For this review, take the finished solid that the model builds, in its own axes (mm). A direction names the side the tool comes from. Coordinates: 2 decimals unless noted, no trailing zeros. Write each loop counter-clockwise with the first axis right and the second up, starting at its lowest first coordinate (ties: lowest second). Pieces come first, ordered by that corner, then holes.
```python
from build123d import *

# Parameters (mm, degrees)
F1_DEPTH = 25.4


with BuildPart() as f1:
    # F0 (on Top) → F1 (new body)
    with BuildSketch(Plane.XY):
        Polygon((-8.610348, -27.288182), (-4.851862, -27.620565), (-4.851862, -13.374916), (-24.708377, -13.374916), (-26.625844, -15.89603), align=None)
        Polygon((-4.851862, -13.374916), (-4.851862, -27.620565), (10.862285, -29.010251), (23.049237, -11.922023), (15.101224, 10.597347), (-5.166208, 12.319417), (-24.708377, -13.374916), align=None)
        Polygon((-30.251862, -13.374916), (-30.251862, -38.774916), (-4.851862, -38.774916), (-4.851862, -27.620565), (-8.610348, -27.288182), (-26.625844, -15.89603), (-24.708377, -13.374916), align=None)
    extrude(amount=F1_DEPTH)


solid = f1.part
```
Q1. For probe 1 along Y at (x, z) = (-26.5, 15.25); probe 2 along X at (y, z) = (-35, 19.5); probe 3 along X at (y, z) = (10, 2.75), list the stretches that pass through material, from the lowest coordinate up.
Ans:
probe 1: y = -38.77 to -13.37
probe 2: x = -30.25 to -4.85
probe 3: x = -6.93 to 15.31
Q2. Add section C-C (x = -12.5). State the section outline as (y, z) points, then the cut area to 3 significant figures.
Ans:
outline: (-38.77, 0) - (2.68, 0) - (2.68, 25.4) - (-38.77, 25.4) - close
area: 1,050 mm2
Q3. Tool access review of faces 4 (the flat face through (-27, -13.375, 13)), 5 (the flat face through (16.87, -20.586, 12.522)): name each direction out of +Z, -Z, +X, -X, +Y, -Y from which nothing blocks a thin tool from reaching the whole face with its end or side.
Ans:
face 4: +Z, -Z, -X, +Y
face 5: +Z, -Z, +X, -Y
Q4. Add section B-B (y = -30). State the section outline as (x, z) points.
Ans:
outline: (-30.25, 0) - (-4.85, 0) - (-4.85, 25.4) - (-30.25, 25.4) - close
Q5. Add section A-A (z = 9). State the section outline as (x, y) points.
Ans:
outline: (-30.25, -38.77) - (-4.85, -38.77) - (-4.85, -27.62) - (10.86, -29.01) - (23.05, -11.92) - (15.1, 10.6) - (-5.17, 12.32) - (-24.71, -13.37) - (-30.25, -13.37) - close
Q6. Draft analysis for pull direction X (two halves, no side actions). For faces 1 (the flat face through (-14.8, -0.35, 12.52)), 2 (the flat face through (-18, -38.775, 13)), 3 (the flat face through (2.895, -28.306, 12.522)), state which applies: +X half, -X half, draft (parallel to the pull), parting line (faces both ways), or undercut.
Ans:
face 1: -X half
face 2: draft
face 3: undercut
Q7. Clearance check with flat-ended pins moving along their axes: pin 1 Ø5 at (y, z) = (-13.5, 4.5) entering from +X; pin 2 Ø3.5 at (y, z) = (-32, 14.5) entering from +X; pin 3 Ø1.7 at (x, z) = (-27.5, 6.5) entering from +Y; pin 4 Ø1 at (x, y) = (-12.5, 5.5) entering from +Z. State where each tip first meets the part, or that it passes through.
Ans:
pin 1: stops at x = 23.05
pin 2: stops at x = -4.85
pin 3: stops at y = -13.37
pin 4: passes through
